Could you check a few things on this model? Use its own coordinates, in mm. Give positions to 0.01 mm unless a question says otherwise; leave off trailing zeros. Order: outer loops, then holes, each group sorted by start corner. A loop starts at its lowest first (then second) coordinate and runs counter-clockwise, first axis right, second up. Notation, with made-up numbers: (84, 47.5) -> (115, 47.5) arc R22 ccw to (115, 70.5) -> close; hole circle Ø3 at (10, 8). An arc over 180 degrees is marked (long way). Write each question's results on one line, items separated by ' | '.
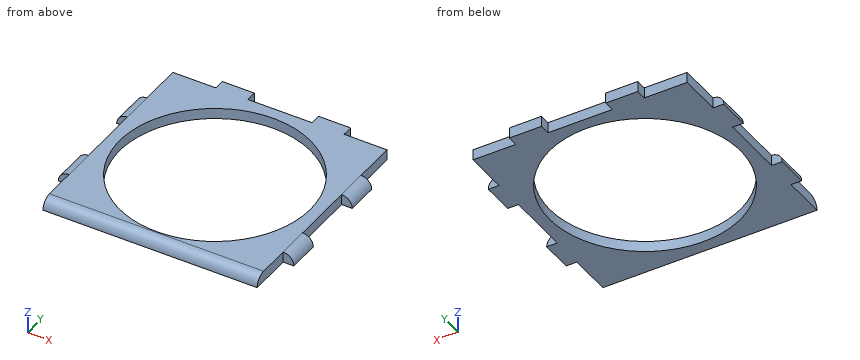
```python
from build123d import *

# Parameters (mm, degrees)
F0_R     = 44.5
F1_DEPTH = 5
F2_R     = 4.99999


# Not quite as in the source:
# - a fillet or chamfer is up to 0.001 mm smaller than in the source, because OpenCascade refuses the exact size


with BuildPart() as f1:
    # F0 (on Top) → F1 (new body)
    with BuildSketch(Plane.XY):
        Polygon((-30, 50), (-50, 50), (-50, 30), (-55, 30), (-55, 15), (-50, 15), (-50, -15), (-55, -15), (-55, -30), (-50, -30), (-50, -50), (50, -50), (50, -30), (55, -30), (55, -15), (50, -15), (50, 15), (55, 15), (55, 30), (50, 30), (50, 50), (30, 50), (30, 55), (15, 55), (15, 50), (-15, 50), (-15, 55), (-30, 55), align=None)
        Circle(F0_R, mode=Mode.SUBTRACT)
    extrude(amount=F1_DEPTH)

    # F2 (radius 5 in the source; OpenCascade refuses exactly that, so slightly less here)
    f2_edges = [f1.edges().sort_by_distance(p)[0] for p in [
        (0, -50, 5),
        (55, -22.5, 5),
        (55, 22.5, 5),
        (-55, 22.5, 5),
        (-55, -22.5, 5),
    ]]
    fillet(f2_edges, radius=F2_R)


solid = f1.part
```
Q1. Suppose I cut it at B-B on y = 0. Please give me the cut outline in (x, z).
Here are the results:
outline: (-50, 0) -> (-44.5, 0) -> (-44.5, 5) -> (-50, 5) -> close; (44.5, 0) -> (50, 0) -> (50, 5) -> (44.5, 5) -> close
Q2. I'm going to push flat-ended pins straight in: pin 1 Ø1.5 at (x, z) = (-23.5, 2) entering from -Y; pin 2 Ø1.5 at (x, z) = (-44, 3.5) entering from +Y; pin 3 Ø1.5 at (y, z) = (53.5, 2.5) entering from +X. Where does each tip first touch, or does it pass through?
Here are the results:
pin 1: stops at y = -49.84 | pin 2: stops at y = 50 | pin 3: stops at x = 30
Q3. I need wall thicknesses on line 1 along Y through (x, z) = (12, 1.45); line 2 along Y through (x, z) = (0, 2.8); line 3 along X through (y, z) = (-38.5, 2). Which ranges of each line are inside material? Lowest first, please.
Here are the results:
line 1: y = -49.79 to -42.85, 42.85 to 50 | line 2: y = -49.14 to -44.5, 44.5 to 50 | line 3: x = -50 to -22.32, 22.32 to 50
